```python
from build123d import *

# Parameters (mm, degrees)
SKETCH1_W           = 117.1702
SKETCH1_H           = 77.0636
SKETCH1_R           = 1.0922
SKETCH1_R_2         = 0.79375
SKETCH1_R_3         = 1.7145
SKETCH1_R_4         = 1.659299133
BOSS_EXTRUDE1_DEPTH = 1.5875


with BuildPart() as part:
    # Sketch1 → Boss-Extrude1 (new body)
    with BuildSketch(Plane.XY):
        with Locations((52.2351, 38.5318)):
            Rectangle(SKETCH1_W, SKETCH1_H)
        with Locations((-3.175, 6.35)):
            Circle(SKETCH1_R, mode=Mode.SUBTRACT)
        with Locations((10.3251, 2.6924)):
            Circle(SKETCH1_R_2, mode=Mode.SUBTRACT)
        with Locations((23.2791, 2.6924)):
            Circle(SKETCH1_R_2, mode=Mode.SUBTRACT)
        with Locations((18.3261, 10.9093)):
            Circle(SKETCH1_R_3, mode=Mode.SUBTRACT)
        with Locations((31.2801, 2.6924)):
            Circle(SKETCH1_R_2, mode=Mode.SUBTRACT)
        with Locations((52.2351, 2.6924)):
            Circle(SKETCH1_R_2, mode=Mode.SUBTRACT)
        with Locations((39.2811, 10.9093)):
            Circle(SKETCH1_R_3, mode=Mode.SUBTRACT)
        with Locations((-3.175, 27.1018)):
            Circle(SKETCH1_R_4, mode=Mode.SUBTRACT)
        with Locations((-3.175, 30.9118)):
            Circle(SKETCH1_R_4, mode=Mode.SUBTRACT)
        with Locations((-3.175, 34.7218)):
            Circle(SKETCH1_R_4, mode=Mode.SUBTRACT)
        with Locations((65.1891, 2.6924)):
            Circle(SKETCH1_R_2, mode=Mode.SUBTRACT)
        with Locations((73.1901, 2.6924)):
            Circle(SKETCH1_R_2, mode=Mode.SUBTRACT)
        with Locations((60.2361, 10.9093)):
            Circle(SKETCH1_R_3, mode=Mode.SUBTRACT)
        with Locations((81.1911, 10.9093)):
            Circle(SKETCH1_R_3, mode=Mode.SUBTRACT)
        with Locations((94.1451, 2.6924)):
            Circle(SKETCH1_R_2, mode=Mode.SUBTRACT)
        with Locations((107.6452, 6.35)):
            Circle(SKETCH1_R, mode=Mode.SUBTRACT)
        with Locations((102.1461, 10.9093)):
            Circle(SKETCH1_R_3, mode=Mode.SUBTRACT)
        with Locations((-3.175, 38.5318)):
            Circle(SKETCH1_R_4, mode=Mode.SUBTRACT)
        with Locations((-3.175, 42.3418)):
            Circle(SKETCH1_R_4, mode=Mode.SUBTRACT)
        with Locations((-3.175, 46.1518)):
            Circle(SKETCH1_R_4, mode=Mode.SUBTRACT)
        with Locations((-3.175, 49.9618)):
            Circle(SKETCH1_R_4, mode=Mode.SUBTRACT)
        with Locations((2.3241, 66.1543)):
            Circle(SKETCH1_R_3, mode=Mode.SUBTRACT)
        with Locations((23.2791, 66.1543)):
            Circle(SKETCH1_R_3, mode=Mode.SUBTRACT)
        with Locations((-3.175, 70.7136)):
            Circle(SKETCH1_R, mode=Mode.SUBTRACT)
        with Locations((10.3251, 74.3712)):
            Circle(SKETCH1_R_2, mode=Mode.SUBTRACT)
        with Locations((18.3261, 74.4347)):
            Circle(SKETCH1_R_2, mode=Mode.SUBTRACT)
        with Locations((44.2341, 66.1543)):
            Circle(SKETCH1_R_3, mode=Mode.SUBTRACT)
        with Locations((31.2801, 74.3712)):
            Circle(SKETCH1_R_2, mode=Mode.SUBTRACT)
        with Locations((52.2351, 74.3712)):
            Circle(SKETCH1_R_2, mode=Mode.SUBTRACT)
        with Locations((65.1891, 66.1543)):
            Circle(SKETCH1_R_3, mode=Mode.SUBTRACT)
        with Locations((86.1441, 66.1543)):
            Circle(SKETCH1_R_3, mode=Mode.SUBTRACT)
        with Locations((60.2361, 74.4347)):
            Circle(SKETCH1_R_2, mode=Mode.SUBTRACT)
        with Locations((73.1901, 74.3712)):
            Circle(SKETCH1_R_2, mode=Mode.SUBTRACT)
        with Locations((107.6452, 70.7136)):
            Circle(SKETCH1_R, mode=Mode.SUBTRACT)
        with Locations((94.1451, 74.3712)):
            Circle(SKETCH1_R_2, mode=Mode.SUBTRACT)
        with Locations((102.1461, 74.4347)):
            Circle(SKETCH1_R_2, mode=Mode.SUBTRACT)
    extrude(amount=BOSS_EXTRUDE1_DEPTH)


solid = part.part
```
Work out the finished part from the listing and answer in its coordinate system (mm). Give positions to 0.01 mm unless a question says otherwise; leave off trailing zeros. Order: outer loops, then holes, each group sorted by start corner. A loop starts at its lowest first (then second) coordinate and runs counter-clockwise, first axis right, second up. Notation, with made-up numbers: (81.5, 33) - (130.5, 33) arc R30 ccw to (130.5, 65) - close; hole circle Ø5 at (-25.75, 20). An arc over 180 degrees is marked (long way). One line per item, written item: value. Start each with the question number.
1. Consider line 1 (Y direction, x = 65.5, z = 1.2); line 2 (Y direction, x = 39.5, z = 1.45); line 3 (X direction, y = 47.5, z = 0.3). Determine where each line is inside the solid, lowest interval first.
2. Each of these flat-tipped pins is pushed along its axis until it touches: pin 1 Ø1.7 at (x, y) = (107.65, 70.71) entering from -Z; pin 2 Ø5.5 at (x, y) = (-3.18, 42.34) entering from +Z. Where does it stop, or does it pass through?
3. Section A-A, the plane x = 2 is taken. Write down the section's boundary in (y, z), then the cut area to 3 significant figures.
4. Section B-B, the plane z = 0.9 is taken. Count the separate pieces of the cut face and the enclosed holes in it, then the cut area to 3 significant figures.
Filled sheet:
1. line 1: 0 to 1.96, 3.42 to 64.47, 67.84 to 77.06
1. line 2: 0 to 9.21, 12.61 to 77.06
1. line 3: -6.35 to -4.14, -2.21 to 110.82
2. pin 1: through
2. pin 2: z = 1.59
3. outline: (0, 0) - (64.47, 0) - (64.47, 1.59) - (0, 1.59) - close; (67.84, 0) - (77.06, 0) - (77.06, 1.59) - (67.84, 1.59) - close
3. area: 117 mm²
4. separate pieces: 1
4. enclosed holes: 36
4. area: 8,830 mm²
